from build123d import *

# Parameters (mm, degrees)
F1_DEPTH = 609.6
F2_W     = 1011.9250416756
F2_H     = 394.0085991383
F3_DEPTH = 76.2
F4_SIZE  = 25.4


with BuildPart() as f1:
    # F0 (on Top) → F1 (new body)
    with BuildSketch(Plane.XY):
        with BuildLine():
            Line((505.9625208378, -720.0900167227), (605.3317958883, -345.9813431194))
            ThreePointArc((605.3317958883, -345.9813431194), (0, -697.23), (-605.3317958883, -345.9813431194))
            Line((-605.3317958883, -345.9813431194), (-505.9625208378, -720.0900167227))
            Line((-505.9625208378, -720.0900167227), (505.9625208378, -720.0900167227))
        make_face()
        with BuildLine():
            Line((605.3317958883, -345.9813431194), (697.23, 0))
            ThreePointArc((697.23, 0), (0, 697.23), (-697.23, 0))
            Line((-697.23, 0), (-605.3317958883, -345.9813431194))
            ThreePointArc((-605.3317958883, -345.9813431194), (0, -697.23), (605.3317958883, -345.9813431194))
        make_face()
    extrude(amount=F1_DEPTH)

    # F2 (on face) → F3 (join)
    with BuildSketch(Plane.XZ.offset(720.0900167227)):
        with Locations((0, 412.5957004309)):
            Rectangle(F2_W, F2_H)
    extrude(amount=F3_DEPTH)

    # F4
    f4_edges = [f1.edges().sort_by_distance(p)[0] for p in [
        (0, -796.290017, 609.6),
        (505.962521, -796.290017, 412.5957),
        (0, -796.290017, 215.591401),
        (-505.962521, -796.290017, 412.5957),
    ]]
    chamfer(f4_edges, length=F4_SIZE)


solid = f1.part
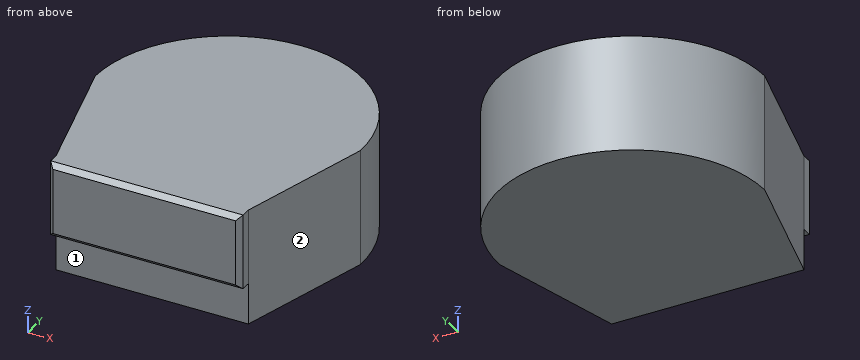
Model file for the job. Use its own axes, mm. Face numbers are marked on the shaded views. A direction names the side the tool comes from. Give positions to 0.01 mm unless a question says otherwise; leave off trailing zeros. Order: outer loops, then holes, each group sorted by start corner. A loop starts at its lowest first (then second) coordinate and runs counter-clockwise, first axis right, second up. Notation, with made-up numbers: (58, 35) - (114, 35) arc R16 ccw to (114, 58) - close; hole circle Ø10 at (53.5, -39). An arc over 180 degrees is marked (long way). Write item = value, one per line. Start each with the question number.
1. Cut at C-C, the plane y = -225. List the corners of the cut face in (x, z).
2. Which spindle directions (+Z, -Z, +X, -X, +Y, -Y) get a long thin tool onto all of the face, cutting with end or side? Do the marked faces 1 and 2. Say none if no direction does.
3. Cut at D-D, the plane z = 117.5. List the corners of the cut face in (x, y).
4. Cut at B-B, the plane x = 0. List the corners of the cut face in (y, z).
5. Drop flat-ended pins along their axis: P1, Ø15, axis at y = -757, z = 382.5, coming from the -X side; P2, Ø12, axis at y = -30, z = 119, coming from the -X side; P3, Ø12, axis at y = 494, z = 443.5, coming from the -X side. Give the stop position or say it passes through.
6. Cut at A-A, the plane z = 348.5. List the corners of the cut face in (x, y), and give its area (3 significant figures).
7. Probe line 1 along X through (y, z) = (-723.5, 238); line 2 along Y through (x, z) = (-273, 90.5); line 3 along X through (y, z) = (525.5, 53.5). List the from-to ranges inside material, lowest first.
Taken from the geometry:
q1.outline = (-637.47, 0) - (637.47, 0) - (637.47, 609.6) - (-637.47, 609.6) - close
q2.face_1 = -Z, +X, -X, -Y
q2.face_2 = +Z, -Z, +X, -Y
q3.outline = (-697.23, 0) - (-505.96, -720.09) - (505.96, -720.09) - (697.23, 0) arc R697.23 ccw to start
q4.outline = (-796.29, 240.99) - (-770.89, 215.59) - (-720.09, 215.59) - (-720.09, 0) - (697.23, 0) - (697.23, 609.6) - (-770.89, 609.6) - (-796.29, 584.2) - close
q5.P1 = -505.96
q5.P2 = -690.86
q5.P3 = -497.98
q6.outline = (-697.23, 0) - (-505.96, -720.09) - (-505.96, -770.89) - (-480.56, -796.29) - (480.56, -796.29) - (505.96, -770.89) - (505.96, -720.09) - (697.23, 0) arc R697.23 ccw to start
q6.area = 1,710,000 mm²
q7.line_1 = -505.96 to 505.96
q7.line_2 = -720.09 to 641.56
q7.line_3 = -458.24 to 458.24
